```python
from build123d import *

# Parameters (mm, degrees)
SKETCH1_R           = 1
BOSS_EXTRUDE1_DEPTH = 1.5
SKETCH2_W           = 30
SKETCH2_H           = 1.5
CUT_EXTRUDE1_DEPTH  = 21.211382931
FILLET1_R           = 1.5


with BuildPart() as part:
    # Sketch1 → Boss-Extrude1 (new body)
    with BuildSketch(Plane.XY):
        with BuildLine():
            Line((-18, 2.5), (18, 2.5))
            ThreePointArc((18, 2.5), (19.414213562, 1.914213562), (20, 0.5))
            Line((20, 0.5), (20, -0.5))
            ThreePointArc((20, -0.5), (19.414213562, -1.914213562), (18, -2.5))
            Line((18, -2.5), (-18, -2.5))
            ThreePointArc((-18, -2.5), (-19.414213562, -1.914213562), (-20, -0.5))
            Line((-20, -0.5), (-20, 0.5))
            ThreePointArc((-20, 0.5), (-19.414213562, 1.914213562), (-18, 2.5))
        make_face()
        with Locations((18, 0)):
            Circle(SKETCH1_R, mode=Mode.SUBTRACT)
        with Locations((-18, 0)):
            Circle(SKETCH1_R, mode=Mode.SUBTRACT)
    extrude(amount=BOSS_EXTRUDE1_DEPTH)

    # Sketch2 → Cut-Extrude1 (cut, through all)
    with BuildSketch(Plane(origin=(0, 0, 0), x_dir=(-1, 0, 0), z_dir=(0, 0, -1))):
        with Locations((0, 2.5)):
            Rectangle(SKETCH2_W, SKETCH2_H)
        with Locations((0, -2.5)):
            Rectangle(SKETCH2_W, SKETCH2_H)
    extrude(amount=-CUT_EXTRUDE1_DEPTH, mode=Mode.SUBTRACT)

    # Fillet1
    # the kernel refuses this fillet: 1.5 mm, written as the material it adds along each edge
    with BuildSketch(Plane(origin=(15, 1.75, 0), x_dir=(0, 1, 0), z_dir=(0, 0, 1)), Plane(origin=(-15, -1.75, 0), x_dir=(0, -1, 0), z_dir=(0, 0, 1))) as fillet1_piece_1:
        with BuildLine():
            CenterArc((1.5, 1.299038106), FILLET1_R, 180, 60)
            Line((0, 1.299038106), (-0.03, 1.299038106))
            Line((-0.03, 1.299038106), (-0.03, 0))
            Line((-0.03, 0), (0, -0.03))
            ThreePointArc((0, -0.03), (0.375, -0.03), (0.735, -0.025980762))
            Line((0.735, -0.025980762), (0.75, 0))
        make_face()
    extrude(amount=1.5)
    with BuildSketch(Plane(origin=(15, -1.75, 0), x_dir=(-1, 0, 0), z_dir=(0, 0, 1))) as fillet1_piece_2:
        with BuildLine():
            CenterArc((1.299038106, 1.5), FILLET1_R, 210, 60)
            Line((0, 0.75), (-0.025980762, 0.735))
            ThreePointArc((-0.025980762, 0.735), (-0.03, 0.375), (-0.03, 0))
            Line((-0.03, 0), (0, -0.03))
            Line((0, -0.03), (1.299038106, -0.03))
            Line((1.299038106, -0.03), (1.299038106, 0))
        make_face()
    extrude(amount=1.5)
    with BuildSketch(Plane(origin=(-15, 1.75, 0), x_dir=(0, 1, 0), z_dir=(0, 0, 1))) as fillet1_piece_3:
        with BuildLine():
            CenterArc((1.5, -1.299038106), FILLET1_R, 120, 60)
            Line((0, -1.299038106), (-0.03, -1.299038106))
            Line((-0.03, -1.299038106), (-0.03, 0))
            Line((-0.03, 0), (0, 0.03))
            ThreePointArc((0, 0.03), (0.375, 0.03), (0.735, 0.025980762))
            Line((0.735, 0.025980762), (0.75, 0))
        make_face()
    extrude(amount=1.5)


solid = part.part
```
Check sheet for the modelled part. Datum: model origin and axes. Units: mm. A direction names the side the tool comes from. Coordinates: 2 decimals unless noted, no trailing zeros. Write each loop counter-clockwise with the first axis right and the second up, starting at its lowest first coordinate (ties: lowest second). Pieces come first, ordered by that corner, then holes. Notation, with made-up numbers: (9, 25.25) -> (58, 25.25) arc R14 ccw to (58, 45.25) -> close; hole circle Ø7 at (-20, 85). An arc over 180 degrees is marked (long way). Use a Markdown table: item, result.
1. Go/stop test with flat-tipped pins: pin 1 Ø0.8 at (x, z) = (3, 0.5) entering from +Y; pin 2 Ø1.2 at (x, y) = (-18, 0) entering from -Z. Record where each tip stops, or that it passes through.
Reported:
| item | result |
|---|---|
| pin 1 | stops at y = 1.75 |
| pin 2 | passes through |
2. Sectioned sample at B-B (z = 0.8). Enter the section's corners in (x, y).
Reported:
| item | result |
|---|---|
| outline | (-20, -0.5) arc R2 ccw to (-18, -2.5) -> (-15, -2.5) arc R1.5 cw to (-13.7, -1.75) -> (13.7, -1.75) arc R1.5 cw to (15, -2.5) -> (18, -2.5) arc R2 ccw to (20, -0.5) -> (20, 0.5) arc R2 ccw to (18, 2.5) -> (15, 2.5) arc R1.5 cw to (13.7, 1.75) -> (-13.7, 1.75) arc R1.5 cw to (-15, 2.5) -> (-18, 2.5) arc R2 ccw to (-20, 0.5) -> close; hole circle Ø2 at (-18, 0); hole circle Ø2 at (18, 0) |
3. Scan lines: line 1 along Y through (x, z) = (18, 0.5); line 2 along X through (y, z) = (0.75, 0.5); line 3 along X through (y, z) = (-0.85, 0.9). Record each from-to range of solid material in increasing order.
Reported:
| item | result |
|---|---|
| line 1 | y = -2.5 to -1, 1 to 2.5 |
| line 2 | x = -19.98 to -18.66, -17.34 to 17.34, 18.66 to 19.98 |
| line 3 | x = -19.97 to -18.53, -17.47 to 17.47, 18.53 to 19.97 |
4. Release check for a two-part mould opening along Y. For faces 4 (the flat face through (16, 2.5, 1)), 5 (the cylindrical face through (14.46, -1.956, 0.74)), 6 (the flat face through (0, 0, 0)), 7 (the cylindrical face through (-19, 0, 1)) record: pulls with the +Y half, pulls with the -Y half, needs draft (parallel to the pull), parting line crosses it, or undercut.
Reported:
| item | result |
|---|---|
| face 4 | pulls with the +Y half |
| face 5 | pulls with the -Y half |
| face 6 | needs draft |
| face 7 | undercut |
5. Sectioned sample at A-A (y = 0). Enter the section's corners in (x, z).
Reported:
| item | result |
|---|---|
| outline | (-20, 0) -> (-19, 0) -> (-19, 1.5) -> (-20, 1.5) -> close; (-17, 0) -> (17, 0) -> (17, 1.5) -> (-17, 1.5) -> close; (19, 0) -> (20, 0) -> (20, 1.5) -> (19, 1.5) -> close |
6. Tool access check on faces 1 (the cylindrical face through (14.441, 1.945, 0.74)), 2 (the cylindrical face through (-19.4, -1.93, 0.74)), 3 (the flat face through (0, -1.75, 1)). Record the directions out of +Z, -Z, +X, -X, +Y, -Y that give a thin tool (end or side, any length) a straight path to the whole face; none if there is none.
Reported:
| item | result |
|---|---|
| face 1 | +Z, -Z, +Y |
| face 2 | +Z, -Z, -X, -Y |
| face 3 | +Z, -Z, -Y |
7. Sectioned sample at C-C (x = 4.5). Enter the section's corners in (y, z).
Reported:
| item | result |
|---|---|
| outline | (-1.75, 0) -> (1.75, 0) -> (1.75, 1.5) -> (-1.75, 1.5) -> close |
8. Sectioned sample at D-D (x = 14.5). Enter the section's corners in (y, z).
Reported:
| item | result |
|---|---|
| outline | (-1.98, 0) -> (1.98, 0) -> (1.98, 1.5) -> (-1.98, 1.5) -> close |
